Study the drawing (mm; zero at the part's minimum x, y, z) and answer. A direction names the side the tool comes from. Coordinates: 2 decimals unless noted, no trailing zeros. Loops run counter-clockwise (first coordinate to the right, second up) from the corner with the lowest first, then second, coordinate; pieces in that order, holes last. Notation, with made-up numbers: (29, 26.25) - (36, 26.25) arc R29 ccw to (36, 59.25) - close; hole circle Ø6 at (58.5, 49). An arc over 180 degrees is marked (long way). Put each result on its own line as item: value.
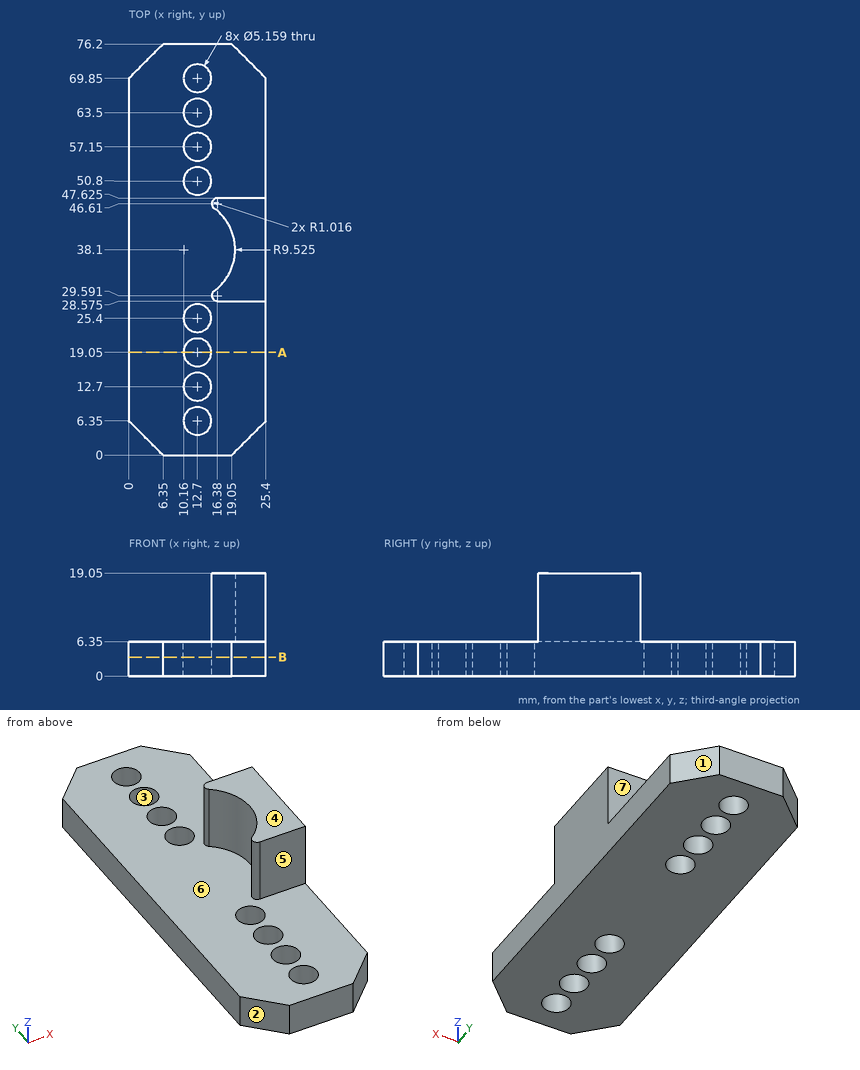
1) Straight lines are drawn through the part: L1, parallel to Z at x = 4, y = 67; L2, parallel to X at y = 5, z = 2; L3, parallel to Y at x = 23.5, z = 11 (1 decimal). For each, find the intervals that lie inside material, in ascending order. Write a range as [from, to].
Found:
L1: z = [0, 6.35]
L2: x = [1.35, 10.5], [14.9, 24.05]
L3: y = [28.6, 47.6]
2) For the marked faces 5, 6 and 7, determine the directions among +Z, -Z, +X, -X, +Y, -Y from which every point of the face is accessible in a straight line to the end or side of a thin tool.
Found:
face 5: +Z, +X, -X, -Y
face 6: +Z, -X
face 7: +Z, +X, -X, +Y
3) The part is cut by section A-A (y = 19.05). Give the vertices of the cut face in (x, z).
Found:
outline: (0, 0) - (10.12, 0) - (10.12, 6.35) - (0, 6.35) - close; (15.28, 0) - (25.4, 0) - (25.4, 6.35) - (15.28, 6.35) - close
4) For a pull along X with two mould halves and no side action, classify the marked faces 1, 2, 3 and 4 as pulls with the +X half, pulls with the -X half, needs draft (parallel to the pull), parting line crosses it, or undercut.
Found:
face 1: pulls with the +X half
face 2: pulls with the -X half
face 3: undercut
face 4: needs draft
5) Each of these flat-tipped pins is pushed along its axis until it touches: pin 1 (7 mm diameter, centred on x = 22.5, z = 11.5, fed in from +Y) (1 decimal); pin 2 (2.5 mm diameter, centred on x = 20, z = 14.5, fed in from -Y) (1 decimal); pin 3 (6 mm diameter, centred on x = 12.7, y = 69.85, fed in from +Z). Where does it stop, or does it pass through?
Found:
pin 1: stops at y = 47.6
pin 2: stops at y = 28.6
pin 3: stops at z = 6.35
6) The part is cut by section B-B (z = 3.5). State how many separate pieces and enclosed holes the cut face has, and give its area (3 significant figures).
Found:
separate pieces: 1
enclosed holes: 8
area: 1,690 mm^2
